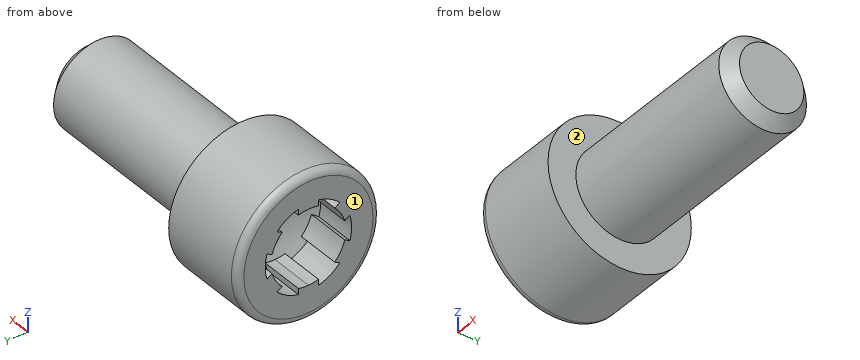
Autodesk Inventor part; units mm, degrees
ref_plane "IDS_WORKPLANE{1}" through (-2.8448, 0, 0) normal (1, 0, 0) x (0, 0, -1)
ref_plane "Work Plane2" through (-1.4224, 0, 0) normal (0, 0, -1) x (1, 0, 0)
ref_plane "YZ Plane" through (0, 0, 0) normal (1, 0, 0) x (0, 1, 0)
sketch "Sketch1" plane through (0, 0, 0) normal (0, 0, 1) x (1, 0, 0)
  line L0 (-2.8448, 0) -> (6.35, 0)
  line L1 (6.35, 0) -> (6.35, 1.4224)
  line L2 (6.35, 1.4224) -> (0, 1.4224)
  line L3 (0, 1.4224) -> (0, 2.3241)
  line L4 (-7.3162, 0) -> (16.036, 0)
  line L5 (0, -0.4648) -> (0, 2.7889)
  line L6 (0, 2.3241) -> (-2.8448, 2.3241)
  line L7 (-2.8448, 0) -> (-2.8448, 2.3241)
  arc A0 (-1.1734, 0) -> (-1.5494, 1.4034) centre (-3.9802, 0) ccw
  line L8 (-2.8448, 1.4034) -> (-1.5494, 1.4034)
  line L9 (12.7, 1.4224) -> (0, 1.4224) construction
  dimension "d0" = 6.35
  dimension "d1" = 2.8448
  dimension "d2" = 2.8448
  dimension "d5" = 4.6482
  dimension "d13" = 2.8068
  dimension "d14" = 2.8068
  dimension "d15" = 1.2954
revolve "Body" add sketch "Sketch1" angle 360 about axis through (-2.8448, 0, 0) along (1, 0, 0) contours A0 L8 L7 L6 L3 L5 L0 | L5 L2 L1 L0
ref_plane "IDS_WORKPLANE{1}" through (-2.8448, 0, 0) normal (1, 0, 0) x (0, 0, -1)
sketch "Sketch2" plane through (-2.8448, 0, 0) normal (1, 0, 0) x (0, 0, -1)
  line L0 (0, -3.6027) -> (0, 5.3473)
  line L1 (5.6384, 0) -> (-3.6512, 0)
  circle A0 centre (0, 0) radius 2.3241
  line L2 (1.3655, 0.3238) -> (1.1714, 0.3239)
  line L3 (0, 0) -> (1.3655, 0.3238) construction
  line L4 (0, 0) -> (4.3113, 4.0687) construction
  line L5 (0, 0) -> (0.4023, 1.3445) construction
  line L6 (0, 0) -> (0.7017, 1.2154) construction
  line L7 (0.4023, 1.3445) -> (0.3053, 1.1764)
  line L8 (0.9632, 1.0207) -> (0.8662, 0.8526)
  line L9 (0, 0) -> (0.9632, 1.0207) construction
  arc A1 (1.2154, 0) -> (1.1714, 0.3239) centre (0, 0) ccw
  arc A2 (0.8662, 0.8526) -> (0.3053, 1.1764) centre (0, 0) ccw
  arc A3 (1.4034, 0) -> (1.3655, 0.3238) centre (0, 0) ccw
  arc A4 (0.9632, 1.0207) -> (0.4023, 1.3445) centre (0, 0) ccw
  arc A5 (1.3655, 0.3238) -> (0.8276, 1.1334) centre (0, 0) ccw construction
  arc A6 (1.1714, 0.3239) -> (0.8662, 0.8526) centre (0, 0) ccw construction
  line L10 (1.3655, -0.3238) -> (1.1714, -0.3239)
  line L11 (0.4023, -1.3445) -> (0.3053, -1.1764)
  line L12 (0.9632, -1.0207) -> (0.8662, -0.8526)
  arc A7 (1.1714, -0.3239) -> (1.2154, 0) centre (0, 0) ccw
  arc A8 (0.3053, -1.1764) -> (0.8662, -0.8526) centre (0, 0) ccw
  arc A9 (1.3655, -0.3238) -> (1.4034, 0) centre (0, 0) ccw
  arc A10 (0.4023, -1.3445) -> (0.9632, -1.0207) centre (0, 0) ccw
  line L13 (-1.3655, 0.3238) -> (-1.1714, 0.3239)
  line L14 (-0.4023, 1.3445) -> (-0.3053, 1.1764)
  line L15 (-0.9632, 1.0207) -> (-0.8662, 0.8526)
  arc A11 (-1.1714, 0.3239) -> (-1.2154, 0) centre (0, 0) ccw
  arc A12 (-0.3053, 1.1764) -> (-0.8662, 0.8526) centre (0, 0) ccw
  arc A13 (-1.3655, 0.3238) -> (-1.4034, 0) centre (0, 0) ccw
  arc A14 (-0.4023, 1.3445) -> (-0.9632, 1.0207) centre (0, 0) ccw
  line L16 (-0.4023, -1.3445) -> (-0.3053, -1.1764)
  arc A15 (-0.8662, -0.8526) -> (-0.3053, -1.1764) centre (0, 0) ccw
  line L17 (-0.9632, -1.0207) -> (-0.8662, -0.8526)
  arc A16 (-0.9632, -1.0207) -> (-0.4023, -1.3445) centre (0, 0) ccw
  arc A17 (-1.2154, 0) -> (-1.1714, -0.3239) centre (0, 0) ccw
  line L18 (-1.3655, -0.3238) -> (-1.1714, -0.3239)
  arc A18 (-1.4034, 0) -> (-1.3655, -0.3238) centre (0, 0) ccw
  point P0 (0.7017, -1.2154)
  point P1 (-0.7017, 1.2154)
  point P2 (-0.7017, -1.2154)
  dimension "d19" = 0.3239
  dimension "d20" = 0.6477
  dimension "d21" = 33.316
  dimension "d22" = 2.8068
  dimension "d23" = 2.4308
extrude "Slot" add sketch "Sketch2" along normal up to next contours A1 L2 A3 L1 | L1 A9 L10 A7 | A17 L18 A18 L1 | L1 A13 L13 A11 | A4 L8 A2 L7 | L11 A8 L12 A10 | L14 A12 L15 A14 | A16 L17 A15 L16
fillet "Fillet1" radius 0.2286 1 edges at (-2.8448, -2.3241, 0)
thread "Thread"
chamfer "Chamfer1" distance 0.3785 distance2 0.3785 1 edges at (6.35, -1.4224, 0) measured on face at (6.35, -0.3549, 0.3144)
ref_plane "Work Plane2" through (-1.4224, 0, 0) normal (0, 0, -1) x (1, 0, 0)
equation "\"d19\" = 0.5 * SBR"
equation "\"d20\" = SBR"
equation "\"d22\" = 1.1547 * SW"
equation "\"d23\" = SW"
equation "\"d17\" = INTI"
equation "\"d24\" = RR"
equation "\"d6\" = GEL"
equation "\"d9\" = -0.5 * SPD + 0.5 * NND"
equation "\"d10\" = GUL"
equation "\"d0\" = NLG"
equation "\"d1\" = KOH"
equation "\"d2\" = NND"
equation "\"d5\" = KOD"
equation "\"d13\" = 1.1547 * SW"
equation "\"d14\" = 1.1547 * SW"
equation "\"d15\" = INTI"
equation "\"NND\" = 2.8448"
equation "\"NLG\" = 6.35"
equation "\"GEL\" = 4.7625"
equation "\"KOD\" = 4.6482"
equation "\"KOH\" = 2.8448"
equation "\"SPD\" = GD1"
equation "\"GUL\" = 0.37846"
equation "\"SBR\" = 0.6477"
equation "\"INTI\" = 1.2954"
equation "\"d11\" = -KOH"
equation "\"SW\" = 2.43078"
equation "\"d16\" = 1.1547 * SW"
equation "\"d18\" = SW"
equation "\"RR\" = 0.2286"
equation "\"TOA\" = 30deg"
equation "\"GD1\" = 2.08788"
equation "\"THREADDIA\" = 2.8448"
equation "\"BDM\" = NND"
equation "\"GD\" = NND"
equation "\"GAL\" = 1.5875"
equation "\"E0\" = 2.86258"
properties part number "ANSI B18.3 - 4-40 UNC - 0.25, SSHCSI" material "Steel, Mild"
Input: part model. Units: mm. Frame: model coordinates. Face numbers are marked on the shaded views. A direction names the side the tool comes from. Give positions to 0.01 mm unless a question says otherwise; leave off trailing zeros. Order: outer loops, then holes, each group sorted by start corner. A loop starts at its lowest first (then second) coordinate and runs counter-clockwise, first axis right, second up. Notation, with made-up numbers: M -27.75,72 L -15.75,72 A20 cw -15.75,91 Z; hole C 70.25,62.5 d1. An arc over 180 degrees is marked long. One line per question, with ' | ' between items. Start each with the question number.
1. First-contact query: pin 1 Ø2 at (x, y) = (1.5, -1) entering from -Z; pin 2 Ø1.5 at (x, z) = (-2, 0.5) entering from -Y. Flat tips, straight axial feed; report the tip coordinate or a pass-through.
2. Material intervals for probe 1 along X at (y, z) = (1.65, 0.8); probe 2 along Z at (x, y) = (0.25, -0.4) (3 decimals); probe 3 along Z at (x, y) = (1.5, 0.55), sorted ascending. Write a range as [from, to].
3. Section query A-A (x = 2.5). Return the cut outline in (y, z), and give its area (3 significant figures).
4. Access query for the marked faces 1 and 2. Directions: +Z, -Z, +X, -X, +Y, -Y. A direction counts if a zero-diameter tool reaches every point of the face in a straight line with its end or side. Return the directions, or none.
Here are the results:
1) pin 1: z = -1.42 | pin 2: y = -2.32
2) probe 1: [-2.84, 0] | probe 2: [-1.365, 1.365] | probe 3: [-1.31, 1.31]
3) outline: C 0,0 d2.84 | area: 6.36 mm²
4) face 1: +Z, -Z, -X, +Y, -Y | face 2: +X
